For this review, use the dimensioned drawing (mm, ordinates from the lowest corner) and the shaded views. A direction names the side the tool comes from. Give positions to 0.01 mm unless a question says otherwise; leave off trailing zeros. Write each loop counter-clockwise with the first axis right and the second up, starting at its lowest first coordinate (ties: lowest second). Pieces come first, ordered by that corner, then holes.
1) Wall thickness on line 1 along X through (y, z) = (3.7, 36.5); line 2 along X through (y, z) = (4.85, 5.5); line 3 along X through (y, z) = (3.35, 28): over which ranges is each line inside the solid? List them lowest first.
2) We need section A-A on z = 5.5. Give the boundary of the cut face in (x, y).
3) We need section D-D on z = 34.5. Give the boundary of the cut face in (x, y).
4) Machinability: for the marked faces 4 and 5, which of the approach directions +Z, -Z, +X, -X, +Y, -Y give a long, thin tool a straight path to every point of the face, cutting with its end or side? Answer none if there is none.
5) Draft analysis for pull direction X (two halves, no side actions). For the marked faces 1, 2 and 3, state which applies: pulls with the +X half, pulls with the -X half, needs draft (parallel to the pull), parting line crosses it, or undercut.
6) We need section C-C on x = 36.5. Give the boundary of the cut face in (y, z).
7) We need section B-B on y = 2.3. Give the boundary of the cut face in (x, z).
8) For P1, Ø1, axis at x = 8.5, y = 2, coming from the -Z side, flat-tipped, find the tip position at first contact; note if it passes through.
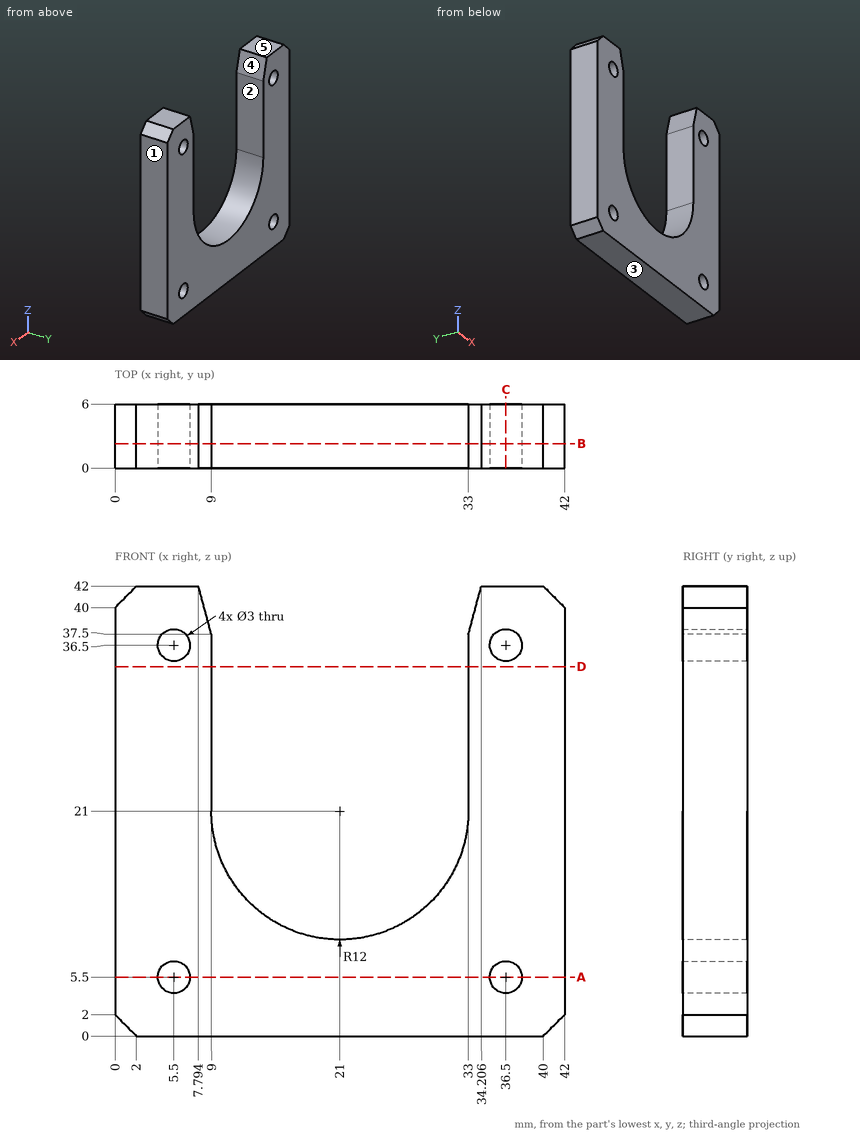
Results list:
1. line 1: x = 0 to 4, 7 to 9, 33 to 35, 38 to 42
1. line 2: x = 0 to 4, 7 to 35, 38 to 42
1. line 3: x = 0 to 9, 33 to 42
2. outline: (0, 0) - (4, 0) - (4, 6) - (0, 6) - close; (7, 0) - (35, 0) - (35, 6) - (7, 6) - close; (38, 0) - (42, 0) - (42, 6) - (38, 6) - close
3. outline: (0, 0) - (9, 0) - (9, 6) - (0, 6) - close; (33, 0) - (42, 0) - (42, 6) - (33, 6) - close
4. face 4: +Z, +Y, -Y
4. face 5: +Z, +X, -X, +Y, -Y
5. face 1: pulls with the +X half
5. face 2: undercut
5. face 3: needs draft
6. outline: (0, 0) - (6, 0) - (6, 4) - (0, 4) - close; (0, 7) - (6, 7) - (6, 35) - (0, 35) - close; (0, 38) - (6, 38) - (6, 42) - (0, 42) - close
7. outline: (0, 2) - (2, 0) - (40, 0) - (42, 2) - (42, 40) - (40, 42) - (34.21, 42) - (33, 37.5) - (33, 21) arc R12 cw to (9, 21) - (9, 37.5) - (7.79, 42) - (2, 42) - (0, 40) - close; hole circle Ø3 at (5.5, 5.5); hole circle Ø3 at (5.5, 36.5); hole circle Ø3 at (36.5, 5.5); hole circle Ø3 at (36.5, 36.5)
8. P1: stops at z = 0
